Input: part model. Units: mm. Frame: model coordinates. Round coordinates to 2 decimals unless told otherwise and drop trailing zeros. Write each loop counter-clockwise with the first axis right and the second up, starting at its lowest first coordinate (ties: lowest second). Pieces come first, ordered by that corner, then holes. Notation, with made-up numbers: M -28.75,-17 L -20.75,-17 A29 ccw -20.75,12 Z; hole C 60,-13 d10. An arc over 180 degrees is marked long. Write each question's results on one line, items separated by ' | '. Start each with the question number.
Autodesk Inventor part; units mm, degrees
ref_plane "YZ Plane" through (0, 0, 0) normal (1, 0, 0) x (0, 1, 0)
ref_plane "XZ Plane" through (0, 0, 0) normal (0, 1, 0) x (-1, 0, 0)
ref_plane "XY Plane" through (0, 0, 0) normal (0, 0, 1) x (1, 0, 0)
sketch "Sketch1" plane through (0, 0, 0) normal (0, 0, 1) x (1, 0, 0)
  circle A0 centre (0, 0) radius 8
  line L0 (1, 7.9373) -> (40.375, 2.9765)
  line L1 (1, -7.9373) -> (40.375, -2.9765)
  line L2 (0, 0) -> (40, 0) construction
  circle A1 centre (40, 0) radius 3
  circle A2 centre (-3.473, -19.6962) radius 5
  line L3 (1.2651, -21.2932) -> (7.5809, -2.5552)
  line L4 (-8.4715, -19.5763) -> (-7.9977, 0.1917)
  line L5 (0, 0) -> (-3.473, -19.6962) construction
  dimension "d0" = 16
  dimension "d1" = 6
  dimension "d2" = 40
  dimension "d3" = 10
  dimension "d4" = 20
  dimension "d5" = 100
extrude "Extrusion1" add sketch "Sketch1" along normal blind 3
fillet "Fillet1" radius 5 1 edges at (5.9783, -7.31, 1.5)
sketch "Sketch2" plane through (0, 0, 3) normal (0, 0, 1) x (1, 0, 0)
  point P0 (0, 0)
  point P1 (0, 0)
hole "Hole1" at (0, 0, 3) direction (0, 0, -1) diameter 6.2 end through all
sketch "Sketch3" plane through (0, 0, 3) normal (0, 0, 1) x (1, 0, 0)
  arc A0 (-8.4715, -19.5763) -> (1.2651, -21.2932) centre (-3.473, -19.6962) ccw
  point P0 (0, 0)
hole "Hole2" at (-3.473, -19.6962, 3) direction (0, 0, -1) diameter 3.4 end through all
properties part number "Pancake_Lever" material "Nylon 6/6"
1. Line query: L1, parallel to X at y = 0, z = 1.2; L2, parallel to Y at x = 0, z = 0.7; L3, parallel to X at y = -20.5, z = 2.85. Output: solid intervals per line, ascending. Write a range as from..to.
2. Cut plane C-C on z = 0.6. Output: boundary loops of the cut face in (x, y) (1 decimal).
3. Cut plane B-B on x = 0. Output: boundary loops of the cut face in (y, z).
4. Cut plane D-D on x = 38.5. Output: boundary loops of the cut face in (y, z).
5. Draft query along X for faces 1 (the face through (11, -4, 3)), 2 (the face through (6.58, -7.984, 1.521)), 3 (the face through (-2.822, -21.267, 1.479)), 4 (the face through (2.75, -1.43, 1.48)). Return one class per face: +X half, -X half, draft (parallel to the pull), parting line (faces both ways), or undercut.
6. Cut plane A-A on y = -2. Output: boundary loops of the cut face in (x, z).
Answers follow:
1) L1: x = -8..-3.1, 3.1..43 | L2: y = -23.29..-3.1, 3.1..8 | L3: x = -8.41..-4.97, -1.98..1.53
2) outline: M -8.5,-19.6 A5 ccw 1.3,-21.3 L 5,-10.3 A5 cw 9.1,-6.9 L 40.4,-3 A3 ccw 40.4,3 L 1,7.9 A8 ccw -8,0.2 Z; hole C -3.5,-19.7 d3.4; hole C 0,0 d6.2
3) outline: M -23.29,0 L -3.1,0 L -3.1,3 L -23.29,3 Z; M 3.1,0 L 8,0 L 8,3 L 3.1,3 Z
4) outline: M -3.21,0 L 3.21,0 L 3.21,3 L -3.21,3 Z
5) face 1: draft | face 2: +X half | face 3: undercut | face 4: undercut
6) outline: M -8.05,0 L -2.37,0 L -2.37,3 L -8.05,3 Z; M 2.37,0 L 42.24,0 L 42.24,3 L 2.37,3 Z
